Source: CAD feature listing. Evaluate the final solid. Frame: model axes, mm. Face numbers are marked on the shaded views. A direction names the side the tool comes from. Give positions to 0.01 mm unless a question says otherwise; leave off trailing zeros. Loops run counter-clockwise (first coordinate to the right, second up) from the corner with the lowest first, then second, coordinate; pieces in that order, holes last. Notation, with made-up numbers: (58.25, 24.5) -> (91.25, 24.5) arc R14 cw to (91.25, 42.5) -> close; hole circle Ø8 at (71, 25). An arc over 180 degrees is marked (long way). Return JSON: item names as keys, results as strings. Group by question number.
(1) Draft query along Y for the marked faces 3, 4, 5 and 6. Return one class per face: released by +Y, released by -Y, zero draft, split by the parting line, or undercut.
(2) Cut plane B-B on z = 7. Return loops of the section in (x, y), then the cut area to 3 significant figures.
(3) Access query for the marked faces 1 and 2. Directions: +Z, -Z, +X, -X, +Y, -Y. A direction counts if a zero-diameter tool reaches every point of the face in a straight line with its end or side. Return the directions, or none.
(4) Pin query (flat end, axial travel): pin 1 (0.6 mm diameter, centred on y = -41, z = 23, fed in from +X); pin 2 (6 mm diameter, centred on y = -37.5, z = 15.5, fed in from +X); pin 3 (19 mm diameter, centred on x = -105.5, y = -22, fed in from +Z). Return the tip coordinate at first contact, or that it passes through.
(5) Cut plane A-A on y = -55. Give the number of separate pieces and of enclosed holes in the cut face, then the cut area to 4 significant figures.
(6) Ray query, line 1 (X direction, y = -24, z = 5.25); line 2 (Y direction, x = -12.5, z = 17.75); line 3 (X direction, y = -19, z = 23.5). Return the intervals inside material, ascending. Write a range as from..to.
(7) Cut plane C-C on x = -106. Return loops of the section in (y, z).
```python
from build123d import *

# Parameters (mm, degrees)
F0_W     = 120
F0_H     = 60
F1_DEPTH = 1.5
F2_DEPTH = 25
F4_DEPTH = 119.25


with BuildPart() as f1:
    # F0 (on Top) → F1 (new body)
    with BuildSketch(Plane.XY):
        with Locations((-60, -30)):
            Rectangle(F0_W, F0_H)
        Polygon((-118.5, -58.5), (-118.5, -30), (-118.5, -1.5), (-80.5, -1.5), (-80.5, -58.5), align=None, mode=Mode.SUBTRACT)
        Polygon((-41, -58.5), (-60, -58.5), (-79, -58.5), (-79, -1.5), (-60, -1.5), (-41, -1.5), align=None, mode=Mode.SUBTRACT)
        Polygon((-1.5, -1.5), (-1.5, -30), (-1.5, -58.5), (-39.5, -58.5), (-39.5, -1.5), align=None, mode=Mode.SUBTRACT)
        Polygon((-118.5, -1.5), (-118.5, -30), (-118.5, -58.5), (-80.5, -58.5), (-80.5, -1.5), align=None)
        Polygon((-79, -58.5), (-60, -58.5), (-41, -58.5), (-41, -1.5), (-60, -1.5), (-79, -1.5), align=None)
        Polygon((-1.5, -58.5), (-1.5, -30), (-1.5, -1.5), (-39.5, -1.5), (-39.5, -58.5), align=None)
    extrude(amount=-F1_DEPTH)

    # F0 (on Top) → F2 (join)
    with BuildSketch(Plane.XY):
        with Locations((-60, -30)):
            Rectangle(F0_W, F0_H)
        Polygon((-118.5, -58.5), (-118.5, -30), (-118.5, -1.5), (-80.5, -1.5), (-80.5, -58.5), align=None, mode=Mode.SUBTRACT)
        Polygon((-41, -58.5), (-60, -58.5), (-79, -58.5), (-79, -1.5), (-60, -1.5), (-41, -1.5), align=None, mode=Mode.SUBTRACT)
        Polygon((-1.5, -1.5), (-1.5, -30), (-1.5, -58.5), (-39.5, -58.5), (-39.5, -1.5), align=None, mode=Mode.SUBTRACT)
    extrude(amount=F2_DEPTH)

    # F3 (on Right) → F4 (cut)
    with BuildSketch(Plane.YZ):
        Polygon((-0.75, 23.390348), (-0.75, 24.390348), (-59.25, 24.390348), (-59.25, 23.390348), (-59.25, 22.390348), (-0.75, 22.390348), align=None)
    extrude(amount=-F4_DEPTH, mode=Mode.SUBTRACT)


solid = f1.part
```
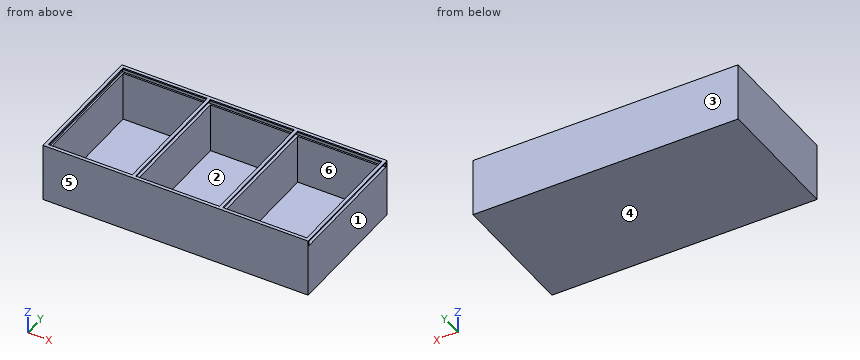
Answers:
{
 "1": {"face 3": "released by +Y", "face 4": "zero draft", "face 5": "released by -Y", "face 6": "undercut"},
 "2": {"outline": "(-120, -60) -> (0, -60) -> (0, 0) -> (-120, 0) -> close; hole (-118.5, -58.5) -> (-80.5, -58.5) -> (-80.5, -1.5) -> (-118.5, -1.5) -> close; hole (-79, -58.5) -> (-41, -58.5) -> (-41, -1.5) -> (-79, -1.5) -> close; hole (-39.5, -58.5) -> (-1.5, -58.5) -> (-1.5, -1.5) -> (-39.5, -1.5) -> close", "area": "702 mm²"},
 "3": {"face 1": "+Z, -Z, +X, +Y, -Y", "face 2": "+Z"},
 "4": {"pin 1": "x = -119.25", "pin 2": "x = 0", "pin 3": "z = 0"},
 "5": {"separate pieces": "4", "enclosed holes": "0", "area": "319.5 mm²"},
 "6": {"line 1": "-120..-118.5, -80.5..-79, -41..-39.5, -1.5..0", "line 2": "-60..-58.5, -1.5..0", "line 3": "-120..-119.25"},
 "7": {"outline": "(-60, -1.5) -> (0, -1.5) -> (0, 25) -> (-1.5, 25) -> (-1.5, 24.39) -> (-0.75, 24.39) -> (-0.75, 22.39) -> (-1.5, 22.39) -> (-1.5, 0) -> (-58.5, 0) -> (-58.5, 22.39) -> (-59.25, 22.39) -> (-59.25, 24.39) -> (-58.5, 24.39) -> (-58.5, 25) -> (-60, 25) -> close"}
}
